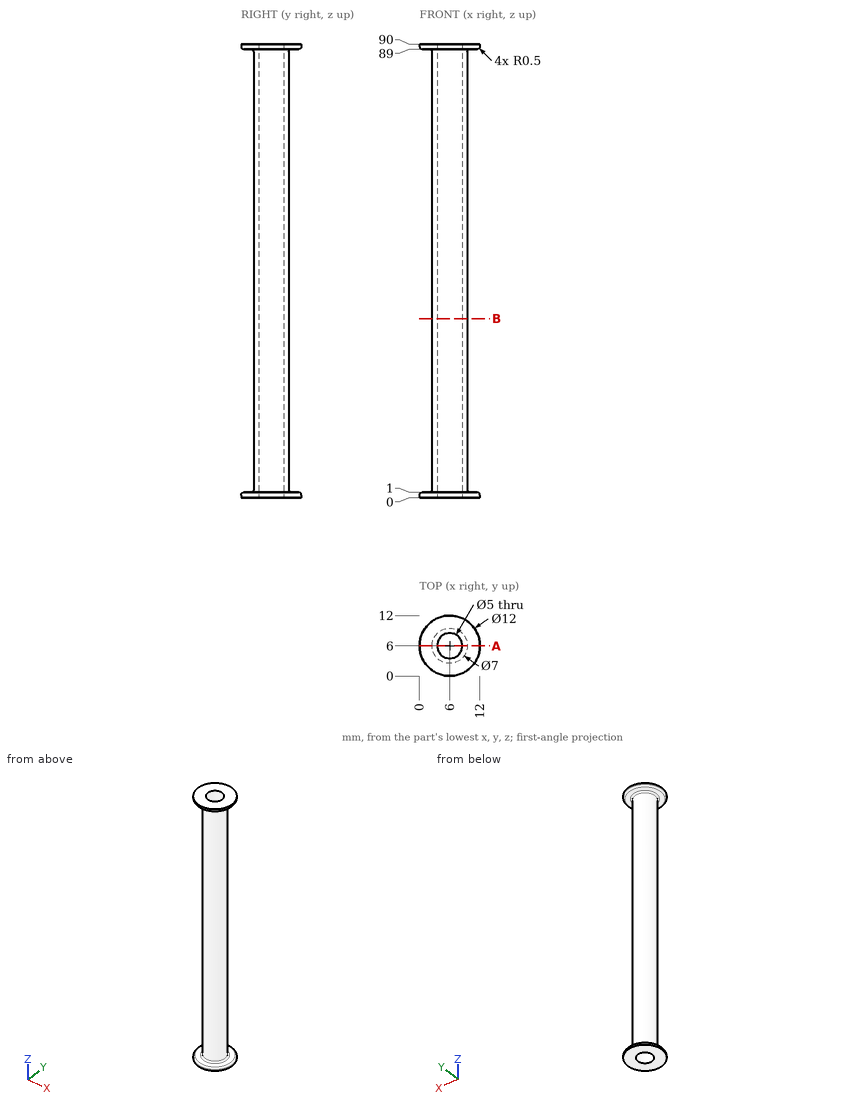
Could you check a few things on this drawing? It's one solid part, dimensions in mm from its lowest x, y, z. Give positions to 0.01 mm unless a question says otherwise; leave off trailing zeros. Order: outer loops, then holes, each group sorted by start corner. A loop starts at its lowest first (then second) coordinate and runs counter-clockwise, first axis right, second up. Notation, with made-up numbers: (-10, 56) - (18, 56) arc R21 ccw to (18, 93) - close; hole circle Ø1 at (-15.75, -25.75). An arc over 180 degrees is marked (long way). One line per item, written item: value. Start each with the question number.
1. For P1, Ø6, axis at y = 2.5, z = 57.5, coming from the -X side; P2, Ø1.5, axis at x = 6, z = 30, coming from the +Y side, each with a flat end and sliding along its axis, tell me the tip position at first contact or that it passes through.
2. If I drill on probe 1 along Z at (x, y) = (1, 8.5); probe 2 along Y at (x, z) = (5.75, 12); probe 3 along Y at (x, z) = (7, 7), over which ranges is the centre line in solid material (lowest first)?
3. Imagine slicing it at B-B on z = 35.5. List the corners of the cut face in (x, y) for me.
4. Imagine slicing it at A-A on y = 6. List the corners of the cut face in (x, z) for me, plus the area to 3 significant figures.
Values:
1. P1: x = 2.54
1. P2: y = 9.5
2. probe 1: 0 to 0.99, 89.01 to 90
2. probe 2: 2.51 to 3.51, 8.49 to 9.49
2. probe 3: 2.65 to 3.71, 8.29 to 9.35
3. outline: circle Ø7 at (6, 6); hole circle Ø5 at (6, 6)
4. outline: (0, 0) - (3.5, 0) - (3.5, 90) - (0, 90) - (0, 89.5) arc R0.5 ccw to (0.5, 89) - (2, 89) arc R0.5 cw to (2.5, 88.5) - (2.5, 1.5) arc R0.5 cw to (2, 1) - (0.5, 1) arc R0.5 ccw to (0, 0.5) - close; (8.5, 0) - (12, 0) - (12, 0.5) arc R0.5 ccw to (11.5, 1) - (10, 1) arc R0.5 cw to (9.5, 1.5) - (9.5, 88.5) arc R0.5 cw to (10, 89) - (11.5, 89) arc R0.5 ccw to (12, 89.5) - (12, 90) - (8.5, 90) - close
4. area: 190 mm²
